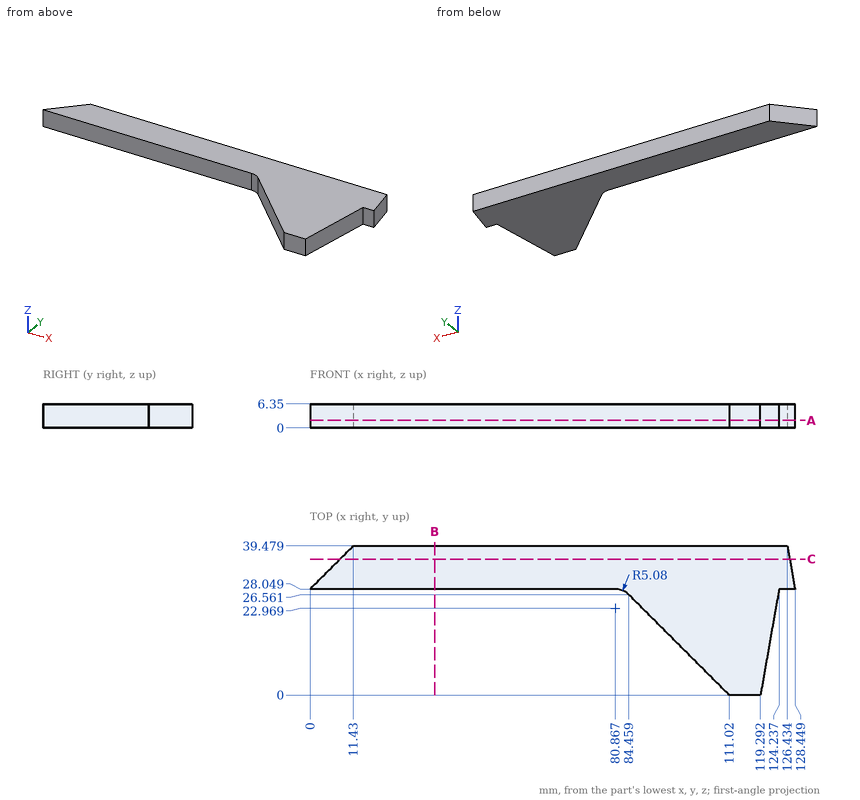
Check sheet for the drawn part. Datum: minimum x, y, z corner. Units: mm. Round coordinates to 2 decimals unless told otherwise and drop trailing zeros. Order: outer loops, then holes, each group sorted by start corner. A loop starts at its lowest first (then second) coordinate and runs counter-clockwise, first axis right, second up. Notation, with made-up numbers: (58.5, 60.5) - (73.5, 60.5) arc R20 cw to (73.5, 97.5) - close; hole circle Ø1 at (-35, -3). An arc over 180 degrees is marked (long way). Use a Markdown table: item, result. Add a question column.
(1) Sectioned sample at A-A, the plane z = 2. Enter the section's corners in (x, y), and give its area (3 significant figures).
(2) Material ranges on line 1 along Y through (x, z) = (14, 4); line 2 along X through (y, z) = (5.5, 5.5); line 3 along Y through (x, z) = (111, 5), recorded low to high. Write a range as [from, to].
(3) Depth check by flat-ended pin: pin 1 (1.3 mm diameter, centred on x = 126.5, z = 4, fed in from -Y); pin 2 (2 mm diameter, centred on x = 95.5, z = 3.5, fed in from -Y); pin 3 (1.5 mm diameter, centred on y = 12.5, z = 4, fed in from +X). Enter the tip coordinate at first touch or a pass-through.
(4) Sectioned sample at B-B, the plane x = 33. Enter the section's corners in (y, z).
(5) Sectioned sample at C-C, the plane y = 36. Enter the section's corners in (x, z).
Answers below:
| question | item | result |
|---|---|---|
| 1 | outline | (0, 28.05) - (80.87, 28.05) arc R5.08 cw to (84.46, 26.56) - (111.02, 0) - (119.29, 0) - (124.24, 28.05) - (128.45, 28.05) - (126.43, 39.48) - (11.43, 39.48) - close |
| 1 | area | 2,090 mm² |
| 2 | line 1 | [28.05, 39.48] |
| 2 | line 2 | [105.52, 120.26] |
| 2 | line 3 | [0.02, 39.48] |
| 3 | pin 1 | y = 28.05 |
| 3 | pin 2 | y = 14.52 |
| 3 | pin 3 | x = 121.63 |
| 4 | outline | (28.05, 0) - (39.48, 0) - (39.48, 6.35) - (28.05, 6.35) - close |
| 5 | outline | (7.95, 0) - (127.05, 0) - (127.05, 6.35) - (7.95, 6.35) - close |
